Read the model definition and answer for the solid it produces. Units are mm, in the model's axes. Face numbers are marked on the shaded views. A direction names the side the tool comes from. Give positions to 0.01 mm unless a question says otherwise; leave off trailing zeros. Order: outer loops, then holes, each group sorted by start corner. A loop starts at its lowest first (then second) coordinate and runs counter-clockwise, first axis right, second up. Notation, with made-up numbers: (-28.75, 85) - (11.25, 85) arc R9 ccw to (11.25, 100) - close; hole circle Ø8 at (-27.75, 3.5). An arc over 180 degrees is marked (long way). Return JSON: item names as keys, results as strings.
```python
from build123d import *

# Parameters (mm, degrees)
F0_W   = 4
F0_H   = 1
F0_W_2 = 1.5
F0_H_2 = 0.5


# Not quite as in the source:
# - a fillet or chamfer that OpenCascade refuses, or shapes differently, is made with other operations: its cross-section is extruded or revolved along the edge and cut away or added


with BuildPart() as f1:
    # F0 (on Front) → F1 (revolve)
    with BuildSketch(Plane.XZ):
        with Locations((-2, -0.5)):
            Rectangle(F0_W, F0_H)
        Polygon((-4, 0), (0, 0), (0, 10), (-4, 10), (-4, 9), (-4, 8.5), align=None)
        with Locations((-4.75, 8.75)):
            Rectangle(F0_W_2, F0_H_2)
        Polygon((-4, 9), (-4, 10), (-11, 10), (-11, 9), (-5.5, 9), align=None)
    revolve(axis=Axis((0, 0, 5), (0, 0, 1)))

    # F2: chamfer of 3 on 1 edges, made by hand

    # F2_s1 → F2_t2 (revolve, cut)
    with BuildSketch(Plane.XZ):
        Polygon((-11, 12), (-8, 9), (-11, 9), align=None)
    revolve(axis=Axis((0, 0, 9), (0, 0, 1)), mode=Mode.SUBTRACT)


solid = f1.part
```
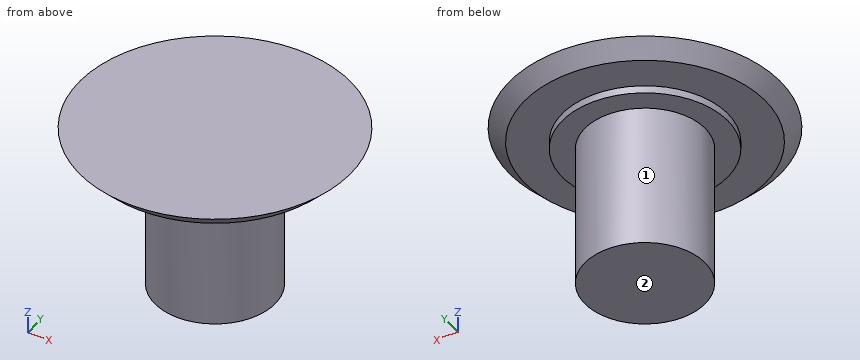
Q1. A cutting plane is placed at C-C (z = 8.75). Write down the section's boundary in (x, y), and give its area (3 significant figures).
Values:
{"outline": "circle Ø11 at (0, 0)", "area": "95.0 mm²"}
Q2. For the marked faces 1 and 2, determine the directions among +Z, -Z, +X, -X, +Y, -Y from which every point of the face is accessible in a straight line to the end or side of a thin tool.
Values:
{"face 1": "-Z", "face 2": "-Z, +X, -X, +Y, -Y"}
Q3. A cutting plane is placed at D-D (z = 6). Write down the section's boundary in (x, y), and give its area (3 significant figures).
Values:
{"outline": "circle Ø8 at (0, 0)", "area": "50.3 mm²"}
Q4. Given pin 1 (1 mm diameter, centred on y = 5, z = 1.5, fed in from -X); pin 2 (1.5 mm diameter, centred on x = 2, z = 4, fed in from -Y), each flat-ended and moving along its own axis, determine where each tip first touches the part or whether it passes through.
Values:
{"pin 1": "passes through", "pin 2": "stops at y = -3.8"}
Q5. Consider L1, parallel to Z at x = 4, y = -5.5; L2, parallel to X at y = 0, z = 4; L3, parallel to X at y = -1.25, z = 9.25. Determine where each line is inside the solid, lowest interval first.
Values:
{"L1": "z = 9 to 10", "L2": "x = -4 to 4", "L3": "x = -8.15 to 8.15"}
Q6. A cutting plane is placed at A-A (x = 0). Write down the section's boundary in (y, z), and give its area (3 significant figures).
Values:
{"outline": "(-9, 10) - (-8, 9) - (-5.5, 9) - (-5.5, 8.5) - (-4, 8.5) - (-4, -1) - (4, -1) - (4, 8.5) - (5.5, 8.5) - (5.5, 9) - (8, 9) - (9, 10) - close", "area": "98.5 mm²"}
